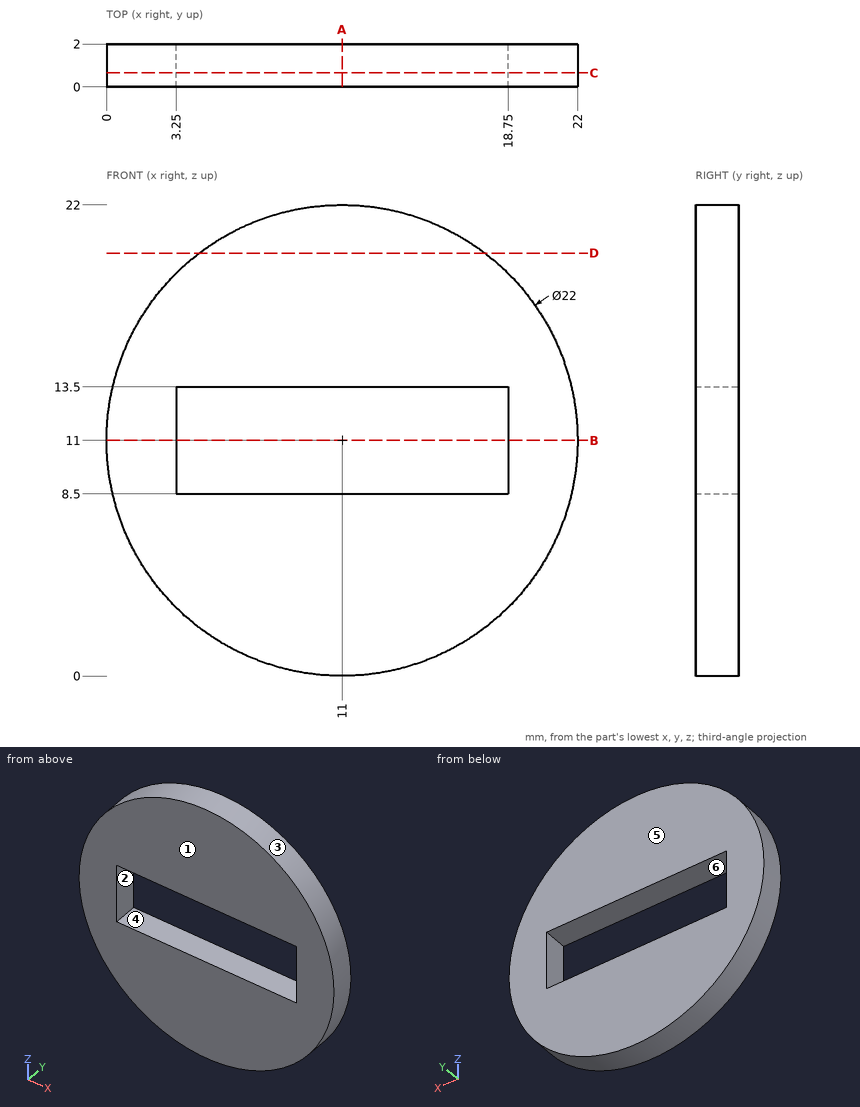
Verification items for this drawing (mm, ordinates from the low corner). A direction names the side the tool comes from. Round coordinates to 2 decimals unless told otherwise and drop trailing zeros. Order: outer loops, then holes, each group sorted by start corner. A loop starts at its lowest first (then second) coordinate and runs counter-clockwise, first axis right, second up. Notation, with made-up numbers: (86, -26) - (131, -26) arc R15 cw to (131, -7) - close; hole circle Ø6 at (-39, 65.5). An arc over 180 degrees is marked (long way). Answer as CSV lines item,"result". Start each with the question number.
1) Section check C-C (y = 0.65). Record the cut outline in (x, z), then the cut area to 3 significant figures.
2) Scan lines: probe 1 along Z at (x, y) = (4, 0.3); probe 2 along Z at (x, y) = (16, 0.6); probe 3 along X at (y, z) = (0.25, 10.5). Record each from-to range of solid material in increasing order.
3) Tool access check on the marked faces 1 and 2. Record the directions out of +Z, -Z, +X, -X, +Y, -Y that give a thin tool (end or side, any length) a straight path to the whole face; none if there is none.
4) Draft check along X on the marked faces 3, 4, 5 and 6. Enter one of: +X half, -X half, draft (parallel to the pull), parting line (faces both ways), or undercut.
5) Section check D-D (z = 19.75). Record the cut outline in (x, y), then the cut area to 3 significant figures.
6) Section check A-A (x = 11). Record the cut outline in (y, z), then the cut area to 3 significant figures.
7) Depth check by flat-ended pin: pin 1 (1 mm diameter, centred on y = 0.5, z = 12, fed in from +X); pin 2 (0.6 mm diameter, centred on x = 10.5, y = 1.5, fed in from -Z). Enter the tip coordinate at first touch or a pass-through.
8) Section check B-B (z = 11). Record the cut outline in (x, y), then the cut area to 3 significant figures.
Determined:
1,outline,"circle Ø22 at (11, 11); hole (3.25, 8.5) - (18.75, 8.5) - (18.75, 13.5) - (3.25, 13.5) - close"
1,area,"303 mm^2"
2,probe 1,"2.51 to 8.5, 13.5 to 19.49"
2,probe 2,"1.2 to 8.5, 13.5 to 20.8"
2,probe 3,"0.01 to 3.25, 18.75 to 21.99"
3,face 1,"+Z, -Z, +X, -X, -Y"
3,face 2,"+Y, -Y"
4,face 3,"parting line"
4,face 4,"undercut"
4,face 5,"draft"
4,face 6,"undercut"
5,outline,"(4.33, 0) - (17.67, 0) - (17.67, 2) - (4.33, 2) - close"
5,area,"26.7 mm^2"
6,outline,"(0, 0) - (2, 0) - (2, 8.5) - (0, 8.5) - close; (0, 13.5) - (2, 13.5) - (2, 22) - (0, 22) - close"
6,area,"34.0 mm^2"
7,pin 1,"x = 21.99"
7,pin 2,"z = 0"
8,outline,"(0, 0) - (3.25, 0) - (3.25, 2) - (0, 2) - close; (18.75, 0) - (22, 0) - (22, 2) - (18.75, 2) - close"
8,area,"13.0 mm^2"
